Check sheet for the modelled part. Datum: model origin and axes. Units: mm. A direction names the side the tool comes from. Round coordinates to 2 decimals unless told otherwise and drop trailing zeros. Loops run counter-clockwise (first coordinate to the right, second up) from the corner with the lowest first, then second, coordinate; pieces in that order, holes last. Notation, with made-up numbers: (7, 78) -> (24, 78) arc R17 ccw to (24, 97) -> close; hole circle Ø8 at (29, 63.5). An arc over 180 degrees is marked (long way). Return JSON: item names as keys, results as strings.
from build123d import *

# Parameters (mm, degrees)
F0_R     = 76.2
F1_DEPTH = 25.4
F3_R     = 5.08
F4_R     = 5.08
F2_R     = 19.05
F5_DEPTH = 12.7
F6_R     = 5.08


with BuildPart() as f1:
    # F0 (on Front) → F1 (new body)
    with BuildSketch(Plane.XZ):
        Circle(F0_R)
    extrude(amount=F1_DEPTH)

    # F3
    f3_edges = [f1.edges().sort_by_distance(p)[0] for p in [
        (-76.2, -25.4, 0),
    ]]
    fillet(f3_edges, radius=F3_R)

    # F4
    f4_edges = [f1.edges().sort_by_distance(p)[0] for p in [
        (76.2, -10.16, 0),
        (-76.2, -20.32, 0),
        (-76.2, 0, 0),
    ]]
    fillet(f4_edges, radius=F4_R)

    # F2 (on face) → F5 (join)
    with BuildSketch(Plane.XZ.offset(25.4)):
        Circle(F2_R)
    extrude(amount=F5_DEPTH)

    # F6
    f6_edges = [f1.edges().sort_by_distance(p)[0] for p in [
        (-19.05, -38.1, 0),
    ]]
    fillet(f6_edges, radius=F6_R)


solid = f1.part
Q1. Section check C-C (y = -11). Record the boundary of the cut face in (x, z), then the cut area to 3 significant figures.
Results list:
{"outline": "circle Ø152.4 at (0, 0)", "area": "18,200 mm^2"}
Q2. Section check B-B (x = 0). Record the boundary of the cut face in (y, z), then the cut area to 3 significant figures.
Results list:
{"outline": "(-38.1, -13.97) arc R5.08 ccw to (-33.02, -19.05) -> (-25.4, -19.05) -> (-25.4, -71.12) arc R5.08 ccw to (-20.32, -76.2) -> (-5.08, -76.2) arc R5.08 ccw to (0, -71.12) -> (0, 71.12) arc R5.08 ccw to (-5.08, 76.2) -> (-20.32, 76.2) arc R5.08 ccw to (-25.4, 71.12) -> (-25.4, 19.05) -> (-33.02, 19.05) arc R5.08 ccw to (-38.1, 13.97) -> close", "area": "4,320 mm^2"}
Q3. Material ranges on line 1 (Y direction, x = 51, z = 18.5); line 2 (X direction, y = -14, z = -1); line 3 (Z direction, x = 17, y = -15), recorded low to high.
Results list:
{"line 1": "-25.4 to 0", "line 2": "-76.19 to 76.19", "line 3": "-74.28 to 74.28"}
Q4. Go/stop test with flat-tipped pins: pin 1 (3 mm diameter, centred on x = -10, y = -25.5, fed in from +Z); pin 2 (3 mm diameter, centred on x = -30, y = -19, fed in from -Z); pin 3 (1.5 mm diameter, centred on x = 38, y = -15, fed in from +Z); pin 4 (1.5 mm diameter, centred on x = -58.5, z = 51.5, fed in from +Y). Record where each tip stops, or that it passes through.
Results list:
{"pin 1": "z = 73.96", "pin 2": "z = -70.67", "pin 3": "z = 66.47", "pin 4": "through"}
Q5. Section check A-A (z = 0). Record the boundary of the cut face in (x, y), then the cut area to 3 significant figures.
Results list:
{"outline": "(-76.2, -20.32) arc R5.08 ccw to (-71.12, -25.4) -> (-19.05, -25.4) -> (-19.05, -33.02) arc R5.08 ccw to (-13.97, -38.1) -> (13.97, -38.1) arc R5.08 ccw to (19.05, -33.02) -> (19.05, -25.4) -> (71.12, -25.4) arc R5.08 ccw to (76.2, -20.32) -> (76.2, -5.08) arc R5.08 ccw to (71.12, 0) -> (-71.12, 0) arc R5.08 ccw to (-76.2, -5.08) -> close", "area": "4,320 mm^2"}
Q6. Tool access check on faces 1 (the flat face through (-1, 0, 1)), 2 (the flat face through (15, -25.4, -15)). Record the directions out of +Z, -Z, +X, -X, +Y, -Y that give a thin tool (end or side, any length) a straight path to the whole face; none if there is none.
Results list:
{"face 1": "+Z, -Z, +X, -X, +Y", "face 2": "-Y"}
